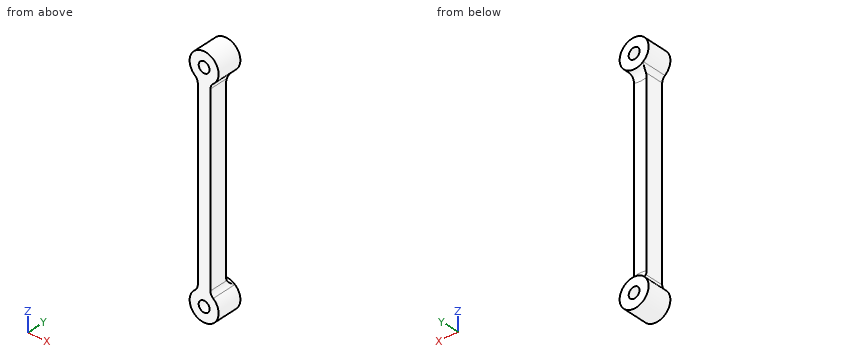
Autodesk Inventor part; units mm, degrees
ref_plane "YZ Plane" through (0, 0, 0) normal (1, 0, 0) x (0, 1, 0)
ref_plane "XZ Plane" through (0, 0, 0) normal (0, 1, 0) x (-1, 0, 0)
ref_plane "XY Plane" through (0, 0, 0) normal (0, 0, 1) x (1, 0, 0)
sketch "Sketch1" plane through (0, 0, 0) normal (0, 1, 0) x (-1, 0, 0)
  circle A0 centre (0, 0) radius 4
  line L0 (0, 0) -> (0, -60)
  circle A1 centre (0, -60) radius 4
  line L1 (0, 0) -> (0, -60) construction
  line L2 (-1.75, 0) -> (-1.75, -60)
  line L3 (1.75, -60) -> (1.75, 0)
  arc A2 (1.75, 0) -> (-1.75, 0) centre (0, 0) ccw
  arc A3 (-1.75, -60) -> (1.75, -60) centre (0, -60) ccw
  point P0 (0, -30)
  point P1 (-1.75, -3.5969)
  point P2 (-1.75, -56.4031)
  point P3 (1.75, -56.4031)
  point P4 (1.75, -3.5969)
  dimension "d0" = 8
  dimension "d1" = 60
  dimension "d2" = 8
  dimension "d3" = 3.5
extrude "Extrusion1" add sketch "Sketch1" along normal blind 7
sketch "Sketch2" plane through (0, 7, 0) normal (0, 1, 0) x (1, 0, 0)
  line L0 (1.75, 3.5969) -> (1.75, 56.4031)
  arc A0 (1.75, 56.4031) -> (-1.75, 56.4031) centre (0, 60) ccw
  line L1 (-1.75, 56.4031) -> (-1.75, 3.5969)
  arc A1 (-1.75, 3.5969) -> (1.75, 3.5969) centre (0, 0) ccw
  circle A2 centre (0, 0) radius 4
  circle A3 centre (0, 60) radius 4
  point P0 (-1.75, 56.4031)
  point P1 (-1.75, 3.5969)
  dimension "d6" = 8
  dimension "d7" = 8
extrude "Extrusion2" cut sketch "Sketch2" against normal blind 2 contours A2 L1 A3 L0
sketch "Sketch3" plane through (0, 7, 0) normal (0, 1, 0) x (1, 0, 0)
  circle A0 centre (0, 0) radius 4
  circle A1 centre (0, 60) radius 4
hole "Hole1" at (0, 7, 0) at (0, 7, -60) direction (0, -1, 0) diameter 3 depth 8
fillet "Fillet1" radius 2 6 edges at (1.75, 2.5, -56.4031) (0, 5, -56) (-1.75, 2.5, -56.4031) (-1.75, 2.5, -3.5969) (0, 5, -4) (1.75, 2.5, -3.5969)
properties part number "leg_link_3_m"
For this review, take the finished solid that the model builds, in its own axes (mm). Coordinates: 2 decimals unless noted, no trailing zeros. Order: outer loops, then holes, each group sorted by start corner. A loop starts at its lowest first (then second) coordinate and runs counter-clockwise, first axis right, second up. Notation, with made-up numbers: (89, 18.25) - (124, 18.25) arc R24 cw to (124, 56.25) - close; hole circle Ø9 at (19, 59.5). An arc over 180 degrees is marked (long way). Use one line per item in the form item = value.
Q1. Consider section D-D (y = 6). Give the boundary of the cut face in (x, z), then the cut area to 3 significant figures.
Checked values:
outline = (-2.5, -56.88) arc R4 ccw (long way) to (2.5, -56.88) arc R2 cw to (1.96, -56.21) arc R4.27 ccw to (-1.96, -56.21) arc R2 cw to start; (-2.5, -3.12) arc R2 cw to (-1.96, -3.79) arc R4.27 ccw to (1.96, -3.79) arc R2 cw to (2.5, -3.12) arc R4 ccw (long way) to start; hole circle Ø3 at (0, -60); hole circle Ø3 at (0, 0)
area = 88.8 mm2
Q2. Consider section A-A (z = -60). Give the boundary of the cut face in (x, y), then the cut area to 3 significant figures.
Checked values:
outline = (-4, 0) - (-1.5, 0) - (-1.5, 7) - (-4, 7) - close; (1.5, 0) - (4, 0) - (4, 7) - (1.5, 7) - close
area = 35.0 mm2
Q3. For probe 1 along Z at (x, y) = (0, 2); probe 2 along X at (y, z) = (1.5, -60); probe 3 along Z at (x, y) = (-0.5, 3.75), list the stretches that pass through material, from the lowest coordinate up. Write a range as from..to.
Checked values:
probe_1 = -64..-61.5, -58.5..-1.5, 1.5..4
probe_2 = -4..-1.5, 1.5..4
probe_3 = -63.97..-61.41, -58.59..-1.41, 1.41..3.97
Q4. For P1, Ø4, axis at x = 0.5, z = -19.5, coming from the +Y side; P2, Ø1, axis at y = 1.5, z = -21.5, coming from the +X side, all flat-tipped, find the tip position at first contact; note any pin that passes through.
Checked values:
P1 = 5
P2 = 1.75
Q5. Consider section C-C (y = 2). Give the boundary of the cut face in (x, z), then the cut area to 3 significant figures.
Checked values:
outline = (-2.5, -56.88) arc R4 ccw (long way) to (2.5, -56.88) arc R2 cw to (1.75, -55.32) - (1.75, -4.68) arc R2 cw to (2.5, -3.12) arc R4 ccw (long way) to (-2.5, -3.12) arc R2 cw to (-1.75, -4.68) - (-1.75, -55.32) arc R2 cw to start; hole circle Ø3 at (0, -60); hole circle Ø3 at (0, 0)
area = 270 mm2
Q6. Consider section B-B (x = 0). Give the boundary of the cut face in (y, z).
Checked values:
outline = (0, -64) - (7, -64) - (7, -61.5) - (0, -61.5) - close; (0, -58.5) - (7, -58.5) - (7, -56) arc R2 cw to (5, -54) - (5, -6) arc R2 cw to (7, -4) - (7, -1.5) - (0, -1.5) - close; (0, 1.5) - (7, 1.5) - (7, 4) - (0, 4) - close
